from build123d import *

# Parameters (mm, degrees)
SKETCH1_R           = 1.5
BOSS_EXTRUDE1_DEPTH = 2
SKETCH1_3_R         = 1.5
BOSS_EXTRUDE2_DEPTH = 8
SKETCH2_R           = 2
CUT_EXTRUDE1_DEPTH  = 10


with BuildPart() as part:
    # Sketch1 → Boss-Extrude1 (new body)
    with BuildSketch(Plane.XY):
        with BuildLine():
            Line((-4.883232135, 1.074264362), (-5, 0))
            ThreePointArc((-5, 0), (0, -5), (5, 0))
            Line((5, 0), (4.883232135, 1.074264362))
            Line((4.883232135, 1.074264362), (2.5, 23))
            ThreePointArc((2.5, 23), (0, 25.5), (-2.5, 23))
            Line((-2.5, 23), (-4.883232135, 1.074264362))
        make_face()
        with Locations((0, 23)):
            Circle(SKETCH1_R, mode=Mode.SUBTRACT)
    extrude(amount=BOSS_EXTRUDE1_DEPTH)

    # Sketch1<3> → Boss-Extrude2 (add)
    with BuildSketch(Plane.XY):
        with Locations((0, 23)):
            Circle(SKETCH1_3_R)
    extrude(amount=BOSS_EXTRUDE2_DEPTH)

    # Sketch2 → Cut-Extrude1 (cut)
    with BuildSketch(Plane.XY.offset(2)):
        Circle(SKETCH2_R)
    extrude(amount=-CUT_EXTRUDE1_DEPTH, mode=Mode.SUBTRACT)


solid = part.part
Part model, mm, in its own coordinate system. A direction names the side the tool comes from. Coordinates: 2 decimals unless noted, no trailing zeros. Loops run counter-clockwise (first coordinate to the right, second up) from the corner with the lowest first, then second, coordinate; pieces in that order, holes last. Notation, with made-up numbers: (87.5, 22.25) -> (105.5, 22.25) arc R27 ccw to (105.5, 56.25) -> close; hole circle Ø7 at (59, 40.25). An arc over 180 degrees is marked (long way). Use a Markdown table: item, result. Add a question column.
Item 1: Which spindle directions (+Z, -Z, +X, -X, +Y, -Y) get a long thin tool onto all of the face, cutting with end or side? Do faces 1 (the cylindrical face through (-0.195, 24.487, 4.958)), 2 (the flat face through (0, 10, 0)). Say none if no direction does.
Item 2: Probe probe 1 along Y at (x, z) = (0, 1.3); probe 2 along Z at (x, y) = (2.25, 21); probe 3 along X at (y, z) = (17, 1). List the from-to ranges inside material, lowest first.
Item 3: Band-saw the part on D-D on z = 5. Write the cut outline in (x, y).
Item 4: Band-saw the part on C-C on y = 22.5. Write the cut outline in (x, z).
Item 5: Band-saw the part on B-B on y = -1. Write the cut outline in (x, z).
Item 6: Pull direction X, two halves, no side cores. Call faces 3 (the cylindrical face through (0, -5, 1)), 4 (the flat face through (0, 7, 2)), 5 (the cylindrical face through (0, -2, 1)): +X half, -X half, draft (parallel to the pull), parting line (faces both ways), or undercut.
Item 7: Band-saw the part on A-A on x = 0. Write the cut outline in (y, z), plus the area to 3 significant figures.
Item 8: Flat gauge pins, fed straight in: P1, Ø3, axis at x = 1.5, z = 5, coming from the +Y side; P2, Ø4, axis at x = 1.5, y = 14, coming from the -Z side; P3, Ø1.5, axis at y = 11.5, z = 1.5, coming from the +X side; P4, Ø1, axis at x = 2.5, z = 7, coming from the -Y side. Where does each tip first touch, or does it go through?
Geometry says:
| question | item | result |
|---|---|---|
| 1 | face 1 | +Z |
| 1 | face 2 | -Z, +X, -X, +Y, -Y |
| 2 | probe 1 | -5 to -2, 2 to 25.5 |
| 2 | probe 2 | 0 to 2 |
| 2 | probe 3 | -3.15 to 3.15 |
| 3 | outline | circle Ø3 at (0, 23) |
| 4 | outline | (-2.55, 0) -> (2.55, 0) -> (2.55, 2) -> (1.41, 2) -> (1.41, 8) -> (-1.41, 8) -> (-1.41, 2) -> (-2.55, 2) -> close |
| 5 | outline | (-4.9, 0) -> (-1.73, 0) -> (-1.73, 2) -> (-4.9, 2) -> close; (1.73, 0) -> (4.9, 0) -> (4.9, 2) -> (1.73, 2) -> close |
| 6 | face 3 | parting line |
| 6 | face 4 | draft |
| 6 | face 5 | undercut |
| 7 | outline | (-5, 0) -> (-2, 0) -> (-2, 2) -> (-5, 2) -> close; (2, 0) -> (25.5, 0) -> (25.5, 2) -> (24.5, 2) -> (24.5, 8) -> (21.5, 8) -> (21.5, 2) -> (2, 2) -> close |
| 7 | area | 71.0 mm² |
| 8 | P1 | y = 24.5 |
| 8 | P2 | z = 0 |
| 8 | P3 | x = 3.83 |
| 8 | P4 | through |
